Geometry check sheet. Reference: the model listing, model coordinates, mm. Give positions to 0.01 mm unless a question says otherwise; leave off trailing zeros. Loops run counter-clockwise (first coordinate to the right, second up) from the corner with the lowest first, then second, coordinate; pieces in that order, holes last. Notation, with made-up numbers: (55, -1) -> (89, -1) arc R22 ccw to (89, 21) -> close; hole circle Ø6 at (14, 8). An arc over 180 degrees is marked (long way). Answer as a JSON object with one key per item and string values.
from build123d import *

# Parameters (mm, degrees)
SKETCH1_W           = 580
SKETCH1_H           = 80
SKETCH1_R           = 12.6
BOSS_EXTRUDE1_DEPTH = 8
SKETCH2_R           = 5
CUT_EXTRUDE1_DEPTH  = 301.93853193


with BuildPart() as part:
    # Sketch1 → Boss-Extrude1 (new, symmetric)
    with BuildSketch(Plane.XY):
        Rectangle(SKETCH1_W, SKETCH1_H)
        with Locations((-240, -20)):
            Circle(SKETCH1_R, mode=Mode.SUBTRACT)
        with Locations((-120, -20)):
            Circle(SKETCH1_R, mode=Mode.SUBTRACT)
        with Locations((0, -20)):
            Circle(SKETCH1_R, mode=Mode.SUBTRACT)
        with Locations((120, -20)):
            Circle(SKETCH1_R, mode=Mode.SUBTRACT)
        with Locations((240, -20)):
            Circle(SKETCH1_R, mode=Mode.SUBTRACT)
    extrude(amount=BOSS_EXTRUDE1_DEPTH, both=True)

    # Sketch2 → Cut-Extrude1 (cut, through all)
    with BuildSketch(Plane(origin=(0, 40, 0), x_dir=(1, 0, 0), z_dir=(0, 1, 0))):
        with Locations(Location((-265, 0, 0), (0, 0, 270))):
            Circle(SKETCH2_R)
        with Locations(Location((265, 0, 0), (0, 0, 270))):
            Circle(SKETCH2_R)
    extrude(amount=-CUT_EXTRUDE1_DEPTH, mode=Mode.SUBTRACT)


solid = part.part
1) Depth check by flat-ended pin: P1, Ø20, axis at x = -240, y = -20, coming from the -Z side. Enter the tip coordinate at first touch or a pass-through.
Geometry check:
{"P1": "passes through"}
2) Section check D-D on y = 1. Record the cut outline in (x, z), plus the area to 3 significant figures.
Geometry check:
{"outline": "(-290, -8) -> (290, -8) -> (290, 8) -> (-290, 8) -> close; hole circle Ø10 at (-265, 0); hole circle Ø10 at (265, 0)", "area": "9,120 mm2"}
3) Draft check along X on faces 1 (the face through (-108.361, -24.826, -0.112)), 2 (the face through (227.412, -19.446, -0.112)), 3 (the face through (-4, 1, 8)), 4 (the face through (-290, -1, 0)). Enter one of: pulls with the +X half, pulls with the -X half, needs draft (parallel to the pull), parting line crosses it, or undercut.
Geometry check:
{"face 1": "undercut", "face 2": "undercut", "face 3": "needs draft", "face 4": "pulls with the -X half"}
4) Material ranges on line 1 along X through (y, z) = (21.5, 0); line 2 along Y through (x, z) = (-240, -0.75); line 3 along X through (y, z) = (-27, -5.5), recorded low to high. Write a range as from..to.
Geometry check:
{"line 1": "x = -290..-270, -260..260, 270..290", "line 2": "y = -40..-32.6, -7.4..40", "line 3": "x = -290..-250.48, -229.52..-130.48, -109.52..-10.48, 10.48..109.52, 130.48..229.52, 250.48..290"}
5) Section check C-C on z = 0. Record the cut outline in (x, y).
Geometry check:
{"outline": "(-290, -40) -> (-270, -40) -> (-270, 40) -> (-290, 40) -> close; (-260, -40) -> (260, -40) -> (260, 40) -> (-260, 40) -> close; (270, -40) -> (290, -40) -> (290, 40) -> (270, 40) -> close; hole circle Ø25.2 at (-240, -20); hole circle Ø25.2 at (-120, -20); hole circle Ø25.2 at (0, -20); hole circle Ø25.2 at (120, -20); hole circle Ø25.2 at (240, -20)"}
6) Section check A-A on y = -20. Record the cut outline in (x, z), plus the area to 3 significant figures.
Geometry check:
{"outline": "(-290, -8) -> (-252.6, -8) -> (-252.6, 8) -> (-290, 8) -> close; (-227.4, -8) -> (-132.6, -8) -> (-132.6, 8) -> (-227.4, 8) -> close; (-107.4, -8) -> (-12.6, -8) -> (-12.6, 8) -> (-107.4, 8) -> close; (12.6, -8) -> (107.4, -8) -> (107.4, 8) -> (12.6, 8) -> close; (132.6, -8) -> (227.4, -8) -> (227.4, 8) -> (132.6, 8) -> close; (252.6, -8) -> (290, -8) -> (290, 8) -> (252.6, 8) -> close; hole circle Ø10 at (-265, 0); hole circle Ø10 at (265, 0)", "area": "7,110 mm2"}
7) Section check B-B on x = 265. Record the cut outline in (y, z).
Geometry check:
{"outline": "(-40, -8) -> (40, -8) -> (40, -5) -> (-40, -5) -> close; (-40, 5) -> (40, 5) -> (40, 8) -> (-40, 8) -> close"}
